Check sheet for the drawn part. Datum: minimum x, y, z corner. Units: mm. Coordinates: 2 decimals unless noted, no trailing zeros. Write each loop counter-clockwise with the first axis right and the second up, starting at its lowest first coordinate (ties: lowest second). Pieces come first, ordered by that corner, then holes. Notation, with made-up numbers: M 10,51.25 L 65,51.25 A25 ccw 65,65.25 Z; hole C 57,-30 d5. An arc over 180 degrees is marked long. Answer as a JSON object with one key per item and string values. Group by question number.
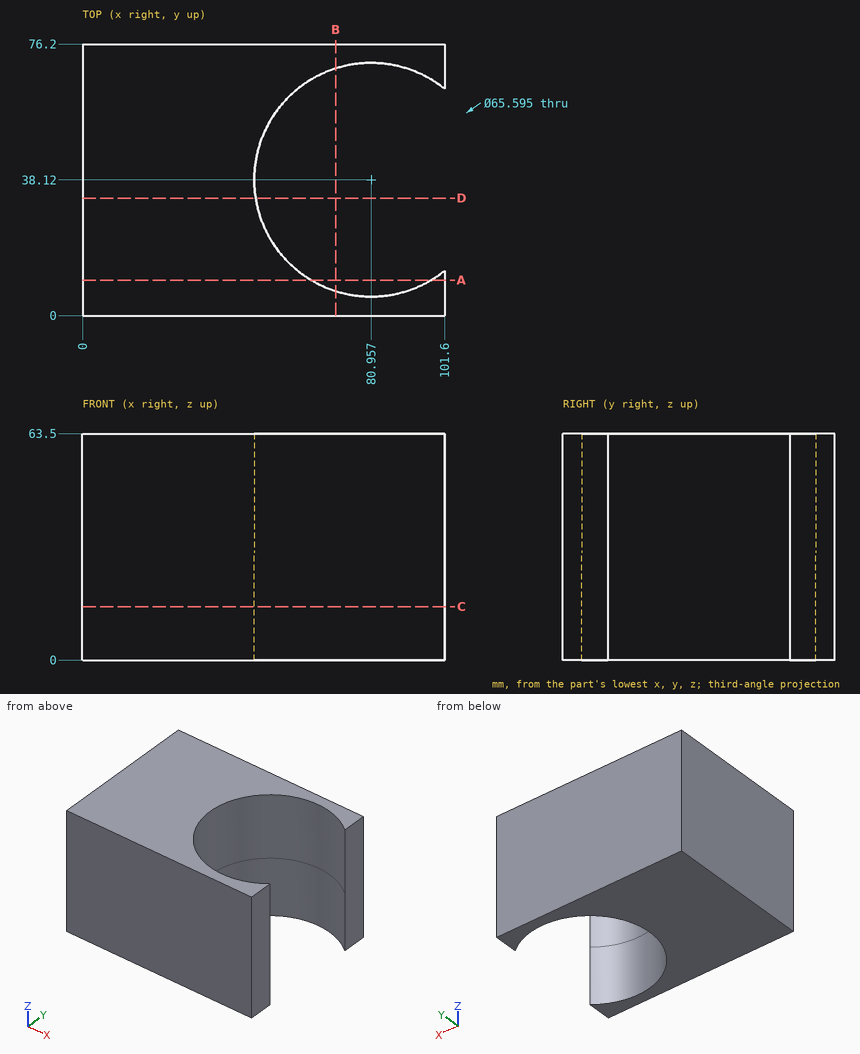
1) Go/stop test with a flat-tipped pin: pin 1 Ø1 at (y, z) = (52.5, 56.5) entering from +X. Record where the tip stops, or that it passes through.
2) Material ranges on probe 1 along Y at (x, z) = (56, 36.5); probe 2 along Y at (x, z) = (91, 20); probe 3 along X at (y, z) = (68, 24.5) (1 decimal), recorded low to high. Write a range as [from, to].
3) Section check D-D (y = 33). Record the cut outline in (x, z).
4) Section check A-A (y = 10). Record the cut outline in (x, z), then the cut area to 3 significant figures.
5) Section check C-C (z = 15). Record the cut outline in (x, y) (1 decimal), then the cut area to 3 significant figures.
6) Section check B-B (x = 71). Record the cut outline in (y, z), then the cut area to 3 significant figures.
Entries:
{
 "1": {"pin 1": "x = 51.73"},
 "2": {"probe 1": "[0, 16.84], [59.4, 76.2]", "probe 2": "[0, 6.9], [69.34, 76.2]", "probe 3": "[0, 67.4], [94.5, 101.6]"},
 "3": {"outline": "M 0,0 L 48.56,0 L 48.56,63.5 L 0,63.5 Z"},
 "4": {"outline": "M 0,0 L 64.08,0 L 64.08,63.5 L 0,63.5 Z; M 97.84,0 L 101.6,0 L 101.6,63.5 L 97.84,63.5 Z", "area": "4,310 mm^2"},
 "5": {"outline": "M 0,0 L 101.6,0 L 101.6,12.6 A32.8 cw long 101.6,63.6 L 101.6,76.2 L 0,76.2 Z", "area": "4,790 mm^2"},
 "6": {"outline": "M 0,0 L 6.87,0 L 6.87,63.5 L 0,63.5 Z; M 69.37,0 L 76.2,0 L 76.2,63.5 L 69.37,63.5 Z", "area": "870 mm^2"}
}
